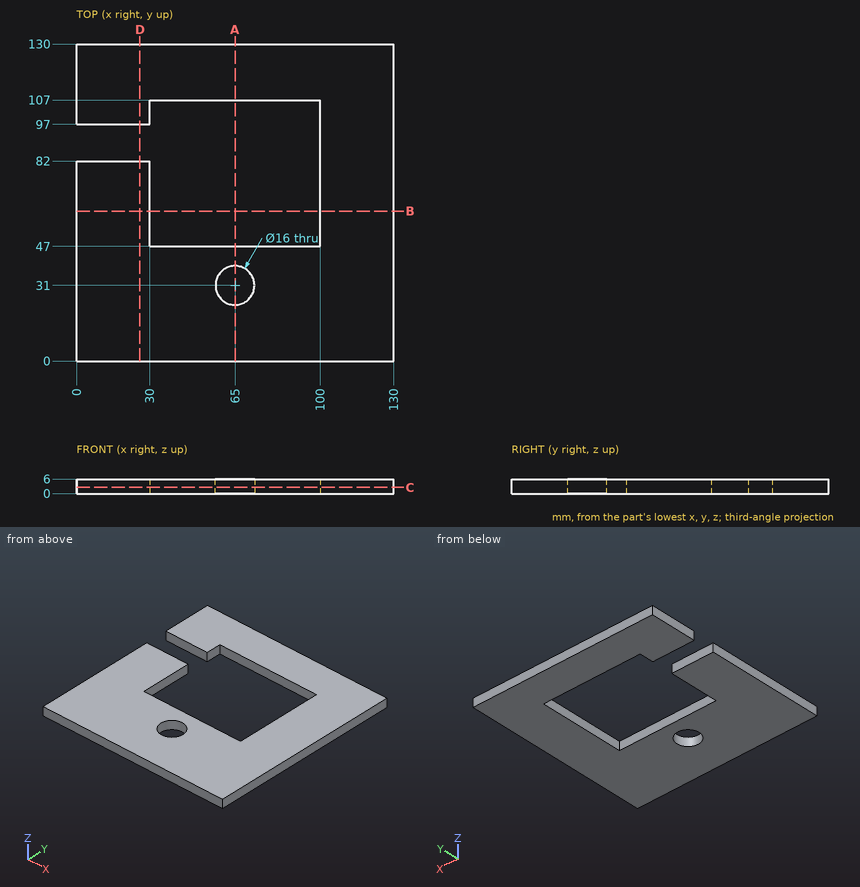
Geometry check sheet. Reference: drawing and pictorial views, mm from the part's lowest x, y, z. Give positions to 0.01 mm unless a question says otherwise; leave off trailing zeros. Loops run counter-clockwise (first coordinate to the right, second up) from the corner with the lowest first, then second, coordinate; pieces in that order, holes last. Notation, with made-up numbers: M -11,80.25 L 42,80.25 A19 ccw 42,103.25 Z; hole C 82.5,75 d2. An arc over 180 degrees is marked long. One line per question, with ' | ' between items.
Item 1: Section check A-A, the plane x = 65. Record the cut outline in (y, z), plus the area to 3 significant figures.
Completed:
outline: M 0,0 L 23,0 L 23,6 L 0,6 Z; M 39,0 L 47,0 L 47,6 L 39,6 Z; M 107,0 L 130,0 L 130,6 L 107,6 Z | area: 324 mm^2
Item 2: Section check B-B, the plane y = 61.5. Record the cut outline in (x, z).
Completed:
outline: M 0,0 L 30,0 L 30,6 L 0,6 Z; M 100,0 L 130,0 L 130,6 L 100,6 Z
Item 3: Depth check by flat-ended pin: P1, Ø9.5, axis at x = 65, y = 31, coming from the +Z side; P2, Ø1.8, axis at x = 72, z = 4.5, coming from the -Y side. Enter the tip coordinate at first touch or a pass-through.
Completed:
P1: passes through | P2: stops at y = 0
Item 4: Section check C-C, the plane z = 2.6. Record the cut outline in (x, y), plus the area to 3 significant figures.
Completed:
outline: M 0,0 L 130,0 L 130,130 L 0,130 L 0,97 L 30,97 L 30,107 L 100,107 L 100,47 L 30,47 L 30,82 L 0,82 Z; hole C 65,31 d16 | area: 12,000 mm^2
Item 5: Thickness scan on line 1 (Y direction, x = 65, z = 1.85); line 2 (X direction, y = 58.5, z = 0.95); line 3 (Y direction, x = 41, z = 1.5). Record the ranges inside material, lowest first. Write a range as [from, to].
Completed:
line 1: y = [0, 23], [39, 47], [107, 130] | line 2: x = [0, 30], [100, 130] | line 3: y = [0, 47], [107, 130]
Item 6: Section check D-D, the plane x = 26. Record the cut outline in (y, z).
Completed:
outline: M 0,0 L 82,0 L 82,6 L 0,6 Z; M 97,0 L 130,0 L 130,6 L 97,6 Z
